Read the model definition and answer for the solid it produces. Units are mm, in the model's axes. A direction names the side the tool comes from. Round coordinates to 2 decimals unless told otherwise and drop trailing zeros. Order: outer loops, then holes, each group sorted by start corner. A loop starts at its lowest first (then second) coordinate and runs counter-clockwise, first axis right, second up. Notation, with made-up numbers: (4, 18.25) - (23, 18.25) arc R25 cw to (23, 41.25) - close; hole circle Ø5 at (-34, -9). An arc over 180 degrees is marked (long way). Put each result on its own line as item: value. Start each with the question number.
Q1. Which of the six approach directions +Z, -Z, +X, -X, +Y, -Y give full straight-line access (tool end or side, diameter ignored) to faces 1 (the face through (0, 0, 0)), 2 (the face through (21.3, 2.4, 15.5)), 3 (the face through (-0.1, 0.5, 14))?
Q2. Section B-B on y = 4 is taken. Give the vertices of the cut face in (x, z).
Q3. Find the intervals of material crossed by line 1 along X through (y, z) = (2.1, 13); line 2 along Y through (x, z) = (4.5, 10.25); line 3 along Z through (x, y) = (0, 0.4), in increasing order. Write a range as from..to.
Q4. Section A-A on x = 7 is taken. Give the vertices of the cut face in (y, z), then the cut area to 3 significant figures.
Q5. Each of these flat-tipped pins is pushed along its axis until it touches: pin 1 Ø10 at (x, z) = (-0.5, 3) entering from +Y; pin 2 Ø2.5 at (y, z) = (3.5, 12.5) entering from -X; pin 3 Ø1 at (y, z) = (2, 10) entering from -X; pin 4 Ø3 at (x, y) = (30.5, 3.5) entering from -Z. Where does it stop, or does it pass through?
Q6. Section C-C on z = 5.25 is taken. Give the vertices of the cut face in (x, y), then the cut area to 3 significant figures.
Autodesk Inventor part; units mm, degrees
ref_plane "YZ Plane" through (0, 0, 0) normal (1, 0, 0) x (0, 1, 0)
ref_plane "XZ Plane" through (0, 0, 0) normal (0, 1, 0) x (-1, 0, 0)
ref_plane "XY Plane" through (0, 0, 0) normal (0, 0, 1) x (1, 0, 0)
sketch "Sketch1" plane through (0, 0, 0) normal (0, 1, 0) x (-1, 0, 0)
  line L0 (6.5, 14) -> (-6.5, 14)
  line L1 (-6.5, 14) -> (-6.5, -14)
  line L2 (-6.5, -14) -> (6.5, -14)
  line L3 (6.5, -14) -> (6.5, 14)
  line L4 (6.5, 14) -> (-6.5, -14) construction
  line L5 (-6.5, 14) -> (6.5, -14) construction
  point P0 (0, 0)
  dimension "d0" = 13
  dimension "d1" = 28
extrude "Extrusion1" add sketch "Sketch1" along normal blind 1
sketch "Sketch2" plane through (6.5, 0, 14) normal (1, 0, 0) x (0, 0, -1)
  circle A0 centre (1, 1.25) radius 0.25
  circle A1 centre (1, 2.5) radius 2.5
  line L0 (0, 1) -> (28, 1)
  line L1 (0, 0) -> (28, 0)
  point P0 (14, 0)
  dimension "d4" = 0.5
  dimension "d5" = 5
  dimension "d6" = 1
extrude "Extrusion2" add sketch "Sketch2" along normal blind 30 contours A0 | A1
properties part number "Telemetrie"
Findings:
1. face 1: +Z, -Z, +X, -X, -Y
1. face 2: +X
1. face 3: +Z, -X, +Y, -Y
2. outline: (6.5, 11) - (36.5, 11) - (36.5, 15) - (6.5, 15) - close
3. line 1: 6.5..36.5
3. line 2: 0..1
3. line 3: -14..14
4. outline: circle Ø5 at (2.5, 13)
4. area: 19.6 mm2
5. pin 1: y = 1
5. pin 2: x = 6.5
5. pin 3: through
5. pin 4: z = 10.5
6. outline: (-6.5, 0) - (6.5, 0) - (6.5, 1) - (-6.5, 1) - close
6. area: 13.0 mm2
